Can you work these out from the model? Positions are in its coordinate system, mm. A direction names the side the tool comes from. Coordinates: 2 decimals unless noted, no trailing zeros. Write each loop counter-clockwise with the first axis right and the second up, starting at its lowest first coordinate (ties: lowest second). Pieces come first, ordered by that corner, then holes. Notation, with made-up numbers: (67, 70.25) - (71, 70.25) arc R13 ccw to (71, 88.25) - close; hole circle Ø3 at (41, 50). An arc over 180 degrees is marked (long way). One line per question, with ' | ' between items. Start each with the question number.
from build123d import *

# Parameters (mm, degrees)
BOSS_EXTRUDE1_DEPTH = 2
SKETCH3_W           = 1.85
SKETCH3_H           = 16
BOSS_EXTRUDE2_DEPTH = 3.1
SKETCH4_W           = 3.35
SKETCH4_H           = 10
BOSS_EXTRUDE3_DEPTH = 2
SKETCH5_W           = 10.9
SKETCH5_H           = 3
BOSS_EXTRUDE4_DEPTH = 2.8
FILLET2_R           = 1
SKETCH7_R           = 1.15
CUT_EXTRUDE2_DEPTH  = 18.740138105
CUT_EXTRUDE3_REACH  = 19.74
SKETCH8_R           = 1.7
FILLET3_START       = -6.300522805
FILLET3_DEPTH       = 1.300522805
FILLET3_START_2     = -8.0000001
FILLET3_2_DEPTH     = 1.699477295
FILLET3_3_DEPTH     = 1.300522805
FILLET3_START_3     = -1.1
FILLET3_4_DEPTH     = 2.1
FILLET3_START_4     = -3.1
FILLET3_5_DEPTH     = 2
FILLET4_R           = 2


with BuildPart() as part:
    # Sketch2 → Boss-Extrude1 (new body)
    with BuildSketch(Plane(origin=(0, 0, 0), x_dir=(1, 0, 0), z_dir=(0, 1, 0))):
        Polygon((9.6, -5), (-9.6, -5), (-9.6, 5), (-9.6, 11), (9.6, 11), (9.6, 5), align=None)
    extrude(amount=BOSS_EXTRUDE1_DEPTH)

    # Sketch3 → Boss-Extrude2 (add)
    with BuildSketch(Plane(origin=(0, 0, 0), x_dir=(1, 0, 0), z_dir=(0, 1, 0))):
        with Locations((-8.675, 3)):
            Rectangle(SKETCH3_W, SKETCH3_H)
        with Locations((8.675, 3)):
            Rectangle(SKETCH3_W, SKETCH3_H)
    extrude(amount=-BOSS_EXTRUDE2_DEPTH)

    # Sketch4 → Boss-Extrude3 (add)
    with BuildSketch(Plane(origin=(0, -3.1, 0), x_dir=(1, 0, 0), z_dir=(0, 1, 0))):
        with Locations((-11.275, 0)):
            Rectangle(SKETCH4_W, SKETCH4_H)
        with Locations((11.275, 0)):
            Rectangle(SKETCH4_W, SKETCH4_H)
    extrude(amount=BOSS_EXTRUDE3_DEPTH)

    # Sketch5 → Boss-Extrude4 (add)
    with BuildSketch(Plane.XZ):
        with Locations((0, 3.5)):
            Rectangle(SKETCH5_W, SKETCH5_H)
    extrude(amount=BOSS_EXTRUDE4_DEPTH)

    # Fillet2
    fillet2_edges = [part.edges().sort_by_distance(p)[0] for p in [
        (-9.6, 2, -3),
        (-7.75, -3.1, -3),
        (7.75, -3.1, -3),
        (9.6, 2, -3),
        (-9.6, -1.1, 0),
        (9.6, -1.1, 0),
        (-5.45, -2.8, 3.5),
        (5.45, -2.8, 3.5),
    ]]
    fillet(fillet2_edges, radius=FILLET2_R)

    # Sketch7 → Cut-Extrude2 (cut, through all)
    with BuildSketch(Plane(origin=(0, 2, 0), x_dir=(1, 0, 0), z_dir=(0, 1, 0))):
        with Locations(Location((-10, 0, 0), (0, 0, 270))):
            Circle(SKETCH7_R)
        with Locations(Location((10, 0, 0), (0, 0, 270))):
            Circle(SKETCH7_R)
    extrude(amount=-CUT_EXTRUDE2_DEPTH, mode=Mode.SUBTRACT)

    # Cut-Extrude3: up to this face of the body (flat: up to its plane)
    cut_extrude3_end = Plane(part.part.faces().sort_by_distance((11.806864318, -1.1, 0))[0])
    # Sketch8 → Cut-Extrude3 (cut, up to the picked face)
    with BuildSketch(Plane(origin=(0, 2, 0), x_dir=(1, 0, 0), z_dir=(0, 1, 0)), mode=Mode.PRIVATE) as cut_extrude3_sk1:
        with Locations((-10, 0)):
            Circle(SKETCH8_R)
    cut_extrude3_tool1 = split(extrude(cut_extrude3_sk1.sketch, amount=-CUT_EXTRUDE3_REACH, mode=Mode.PRIVATE), bisect_by=cut_extrude3_end, keep=Keep.BOTH, mode=Mode.PRIVATE)
    # Sketch8 → Cut-Extrude3 (cut, up to the picked face)
    with BuildSketch(Plane(origin=(0, 2, 0), x_dir=(1, 0, 0), z_dir=(0, 1, 0)), mode=Mode.PRIVATE) as cut_extrude3_sk2:
        with Locations((10, 0)):
            Circle(SKETCH8_R)
    cut_extrude3_tool2 = split(extrude(cut_extrude3_sk2.sketch, amount=-CUT_EXTRUDE3_REACH, mode=Mode.PRIVATE), bisect_by=cut_extrude3_end, keep=Keep.BOTH, mode=Mode.PRIVATE)
    add(cut_extrude3_tool1.solids().sort_by(Axis((-10, 2, 0), (0, -1, 0)))[0], mode=Mode.SUBTRACT)
    add(cut_extrude3_tool2.solids().sort_by(Axis((10, 2, 0), (0, -1, 0)))[0], mode=Mode.SUBTRACT)

    # Fillet3: read off the stored shape, not the designer's step
    # Fillet3 outline → Fillet3 (add)
    with BuildSketch(Plane.XY.offset(FILLET3_START)):
        with BuildLine():
            Line((9.6, -1.1), (10.6, -1.1))
            ThreePointArc((10.6, -1.1), (9.892893219, -0.807106781), (9.6, -0.1))
            Line((9.6, -0.1), (9.6, -1.1))
        make_face()
    extrude(amount=FILLET3_DEPTH)

    # Fillet3 2 outline → Fillet3 2 (add)
    with BuildSketch(Plane.XY.offset(FILLET3_START_2)):
        with BuildLine():
            Line((-9.6, -1.1), (-9.6, -0.1))
            ThreePointArc((-9.6, -0.1), (-9.892893219, -0.807106781), (-10.6, -1.1))
            Line((-10.6, -1.1), (-9.6, -1.1))
        make_face()
        with BuildLine():
            Line((9.6, -1.1), (10.6, -1.1))
            ThreePointArc((10.6, -1.1), (9.892893219, -0.807106781), (9.6, -0.1))
            Line((9.6, -0.1), (9.6, -1.1))
        make_face()
    extrude(amount=FILLET3_2_DEPTH)

    # Fillet3 3 outline → Fillet3 3 (add)
    with BuildSketch(Plane.XY.offset(FILLET3_START)):
        with BuildLine():
            Line((-9.6, -1.1), (-9.6, -0.1))
            ThreePointArc((-9.6, -0.1), (-9.892893219, -0.807106781), (-10.6, -1.1))
            Line((-10.6, -1.1), (-9.6, -1.1))
        make_face()
    extrude(amount=FILLET3_3_DEPTH)

    # Fillet3 4 outline → Fillet3 4 (cut)
    with BuildSketch(Plane(origin=(0, 0, 0), x_dir=(1, 0, 0), z_dir=(0, 1, 0)).offset(FILLET3_START_3)):
        with BuildLine():
            Line((14, 8.0000001), (9.6, 8))
            ThreePointArc((9.6, 8), (10.478679656, 5.878679656), (12.6, 5))
            Line((12.6, 5), (12.95, 5))
            Line((12.95, 5), (14, 5.000000001))
            Line((14, 5.000000001), (14, 8.0000001))
        make_face()
        with BuildLine():
            Line((-12.95, 5), (-12.6, 5))
            ThreePointArc((-12.6, 5), (-10.478679656, 5.878679656), (-9.6, 8))
            Line((-9.6, 8), (-14, 8.0000001))
            Line((-14, 8.0000001), (-14, 5))
            Line((-14, 5), (-12.95, 5))
        make_face()
    extrude(amount=FILLET3_4_DEPTH, mode=Mode.SUBTRACT)

    # Fillet3 5 outline → Fillet3 5 (add)
    with BuildSketch(Plane(origin=(0, 0, 0), x_dir=(1, 0, 0), z_dir=(0, 1, 0)).offset(FILLET3_START_4)):
        with BuildLine():
            ThreePointArc((12.6, 5), (10.478679656, 5.878679656), (9.6, 8))
            Line((9.6, 8), (9.6, 5))
            Line((9.6, 5), (12.6, 5))
        make_face()
        with BuildLine():
            Line((-12.6, 5), (-9.6, 5))
            Line((-9.6, 5), (-9.6, 8))
            ThreePointArc((-9.6, 8), (-10.478679656, 5.878679656), (-12.6, 5))
        make_face()
    extrude(amount=FILLET3_5_DEPTH)

    # Fillet4
    fillet4_edges = [part.edges().sort_by_distance(p)[0] for p in [
        (12.95, -2.1, -5),
        (12.95, -2.1, 5),
        (-12.95, -2.1, -5),
        (-12.95, -2.1, 5),
    ]]
    fillet(fillet4_edges, radius=FILLET4_R)


solid = part.part
(1) If we section it at C-C on y = -1.4: Give the number of separate pieces and of enclosed holes in the cut face, plus the area to 3 significant figures.
(2) Which directions (+Z, -Z, +X, -X, +Y, -Y) give clear straight access to the entire face, cutting with the end or side of a thin tool? Please do faces 1 (the face through (12.95, -2, 0)), 2 (the face through (0, -2.8, 4)), 3 (the face through (-9.6, 0.5, 3.3)).
(3) If we section it at D-D on z = -9: List the corners of the cut face in (x, y) for me.
(4) If we section it at A-A on z = 0: List the corners of the cut face in (x, y) for me.
(5) I'm going to push flat-ended pins straight in: pin 1 (8 mm diameter, centred on x = -4.5, z = -7.5, fed in from -Y); pin 2 (0.9 mm diameter, centred on y = -1, z = 4, fed in from -X); pin 3 (0.8 mm diameter, centred on x = 1, y = -0.5, fed in from -Z). Where does each tip first touch, or does it pass through?
(6) If I drill on probe 1 along X at (y, z) = (-0.05, -8.5); probe 2 along Y at (x, z) = (3, -7); probe 3 along Z at (x, y) = (0, -1.65), over which ranges is the centre line in solid material (lowest first)?
(7) If we mould it in two halves opening along X, with no side actions, what happens to faces 4 (the face through (0, -1, 2)), 5 (the face through (9.6, 0.4, 3.3)), 6 (the face through (0, 0, -5)), 7 (the face through (-9.6, -0.6, -8.3))? For each: +X half, -X half, draft (parallel to the pull), parting line (faces both ways), or undercut.
(8) If we section it at B-B on x = 10: List the corners of the cut face in (y, z) for me, plus the area to 3 significant figures.
Values:
1) separate pieces: 3 | enclosed holes: 2 | area: 152 mm2
2) face 1: +Z, -Z, +X, +Y, -Y | face 2: +Z, -Z, -Y | face 3: +Z, -Z, -X, +Y
3) outline: (-9.6, -3.1) - (-8.75, -3.1) arc R1 ccw to (-7.75, -2.1) - (-7.75, 0) - (7.75, 0) - (7.75, -2.1) arc R1 ccw to (8.75, -3.1) - (9.6, -3.1) - (9.6, 1) arc R1 ccw to (8.6, 2) - (-8.6, 2) arc R1 ccw to (-9.6, 1) - close
4) outline: (-12.95, -3.1) - (-11.15, -3.1) - (-11.15, -1.1) - (-12.95, -1.1) - close; (-8.85, -3.1) - (-8.75, -3.1) arc R1 ccw to (-7.75, -2.1) - (-7.75, 0) - (7.75, 0) - (7.75, -2.1) arc R1 ccw to (8.75, -3.1) - (8.85, -3.1) - (8.85, -1.1) - (8.3, -1.1) - (8.3, 2) - (-8.3, 2) - (-8.3, -1.1) - (-8.85, -1.1) - close; (11.15, -3.1) - (12.95, -3.1) - (12.95, -1.1) - (11.15, -1.1) - close
5) pin 1: y = -3.07 | pin 2: x = -12.87 | pin 3: z = 2
6) probe 1: -9.6 to -7.75, 7.75 to 9.6 | probe 2: 0 to 2 | probe 3: 2 to 5
7) face 4: undercut | face 5: +X half | face 6: undercut | face 7: -X half
8) outline: (-3.1, -6.5) - (-0.9, -6.5) - (-0.9, -1.7) - (-1.1, -1.7) - (-1.1, -1.15) - (-3.1, -1.15) - close; (-3.1, 1.15) - (-1.1, 1.15) - (-1.1, 1.7) - (-0.9, 1.7) - (-0.9, 5) - (-3.1, 5) - close | area: 20.0 mm2
